Here's how the part is built. I have some questions about the finished solid (model axes, mm). Face numbers are marked on the shaded views. A direction names the side the tool comes from. Round coordinates to 2 decimals unless told otherwise and drop trailing zeros. Loops run counter-clockwise (first coordinate to the right, second up) from the corner with the lowest first, then second, coordinate; pieces in that order, holes last. Notation, with made-up numbers: M -18,82 L -7,82 A12 cw -7,89 Z; hole C -19,15 d1. An arc over 180 degrees is marked long. Answer as a JSON object with one key per item and string values.
from build123d import *

# Parameters (mm, degrees)
BOSS_EXTRUDE1_DEPTH = 15
SKETCH3_R           = 37.5
SKETCH3_R_2         = 25
BOSS_EXTRUDE2_DEPTH = 45
CUT_EXTRUDE1_START  = -45
SKETCH4_R           = 25
CUT_EXTRUDE1_DEPTH  = 45


with BuildPart() as part:
    # Sketch1 → Boss-Extrude1 (new body)
    with BuildSketch(Plane(origin=(0, 0, 0), x_dir=(1, 0, 0), z_dir=(0, 1, 0))):
        Polygon((-25, 75), (-25, -75), (-10, -75), (-10, -45), (10, -45), (10, -75), (25, -75), (25, 75), (10, 75), (10, 45), (-10, 45), (-10, 75), align=None)
    extrude(amount=BOSS_EXTRUDE1_DEPTH)

    # Sketch3 → Boss-Extrude2 (add)
    with BuildSketch(Plane.XZ):
        with Locations(Location((0, 0, 0), (0, 0, 270))):
            Circle(SKETCH3_R)
        with Locations(Location((0, 0, 0), (0, 0, 270))):
            Circle(SKETCH3_R_2, mode=Mode.SUBTRACT)
    extrude(amount=-BOSS_EXTRUDE2_DEPTH)

    # Sketch4 → Cut-Extrude1 (cut)
    with BuildSketch(Plane(origin=(0, 15, 0), x_dir=(1, 0, 0), z_dir=(0, 1, 0)).offset(CUT_EXTRUDE1_START)):
        with Locations(Location((0, 0, 0), (0, 0, 90))):
            Circle(SKETCH4_R)
    extrude(amount=CUT_EXTRUDE1_DEPTH, mode=Mode.SUBTRACT)


solid = part.part
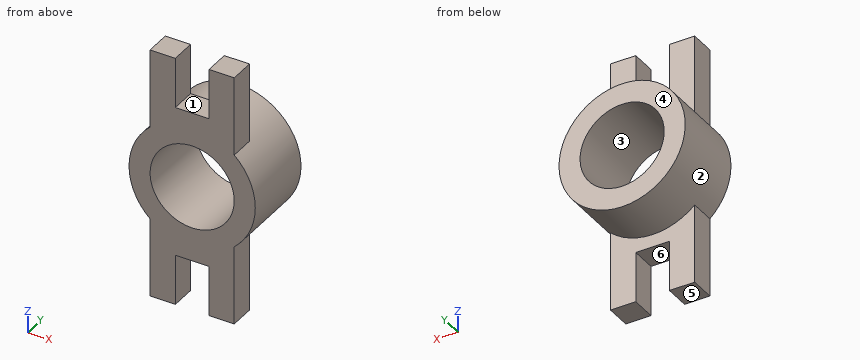
Item 1: If we mould it in two halves opening along X, with no side actions, what happens to the marked faces 1, 2, 3 and 4? For each: pulls with the +X half, pulls with the -X half, needs draft (parallel to the pull), parting line crosses it, or undercut.
Resolved:
{"face 1": "undercut", "face 2": "parting line crosses it", "face 3": "undercut", "face 4": "needs draft"}
Item 2: I want a section at A-A, the plane x = 0. Please give me the cut outline in (y, z), then the cut area to 3 significant figures.
Resolved:
{"outline": "M 0,-45 L 15,-45 L 15,-37.5 L 45,-37.5 L 45,-25 L 0,-25 Z; M 0,25 L 45,25 L 45,37.5 L 15,37.5 L 15,45 L 0,45 Z", "area": "1,350 mm²"}
Item 3: I want a section at C-C, the plane z = -36. Please give me the cut outline in (x, y).
Resolved:
{"outline": "M -25,0 L 25,0 L 25,15 L 10.5,15 L 10.5,45 L -10.5,45 L -10.5,15 L -25,15 Z"}
Item 4: On a 3-axis mill with a long thin cutter (end or side, diameter ignored), from which of +Z, -Z, +X, -X, +Y, -Y can I reach the whole of each face in a straight line? I mean the marked faces 5 and 6. Say none if no direction works.
Resolved:
{"face 5": "-Z, +X, -X, +Y, -Y", "face 6": "-Z, +Y, -Y"}
Item 5: I'm going to push flat-ended pins straight in: pin 1 Ø16.5 at (y, z) = (5.5, -54.5) entering from -X; pin 2 Ø4.5 at (y, z) = (6, -67) entering from +X; pin 3 Ø1 at (x, y) = (14.5, 27) entering from -Z. Where does each tip first touch, or does it pass through?
Resolved:
{"pin 1": "x = -25", "pin 2": "x = 25", "pin 3": "z = -34.79"}
Item 6: I want a section at B-B, the plane z = -13. Please give me the cut outline in (x, y), then the cut area to 3 significant figures.
Resolved:
{"outline": "M -35.17,0 L -21.35,0 L -21.35,45 L -35.17,45 Z; M 21.35,0 L 35.17,0 L 35.17,45 L 21.35,45 Z", "area": "1,240 mm²"}
Item 7: I want a section at D-D, the plane y = 17. Please give me the cut outline in (x, z).
Resolved:
{"outline": "C 0,0 d75; hole C 0,0 d50"}
Item 8: Please list where these lines run through material, in increasing order: probe 1 along X at (y, z) = (7, 46); probe 2 along X at (y, z) = (21, 0); probe 3 along Y at (x, z) = (19.5, 36.5). Write a range as from..to.
Resolved:
{"probe 1": "-25..-10, 10..25", "probe 2": "-37.5..-25, 25..37.5", "probe 3": "0..15"}
